from build123d import *

# Parameters (mm, degrees)
CROQUIS1_W              = 60
CROQUIS1_H              = 62
CROQUIS1_R              = 1.5
SALIENTE_EXTRUIR1_DEPTH = 2
REDONDEO1_R             = 4
CROQUIS3_R              = 1.5
CORTAR_EXTRUIR1_DEPTH   = 2


with BuildPart() as part:
    # Croquis1 → Saliente-Extruir1 (new body)
    with BuildSketch(Plane.XY):
        Rectangle(CROQUIS1_W, CROQUIS1_H)
        with Locations((-25, -26)):
            Circle(CROQUIS1_R, mode=Mode.SUBTRACT)
        with Locations((25, -26)):
            Circle(CROQUIS1_R, mode=Mode.SUBTRACT)
        with Locations((25, 26)):
            Circle(CROQUIS1_R, mode=Mode.SUBTRACT)
        with Locations((-25, 26)):
            Circle(CROQUIS1_R, mode=Mode.SUBTRACT)
    extrude(amount=SALIENTE_EXTRUIR1_DEPTH)

    # Redondeo1
    redondeo1_edges = [part.edges().sort_by_distance(p)[0] for p in [
        (-30, -31, 1),
        (-30, 31, 1),
        (30, 31, 1),
        (30, -31, 1),
    ]]
    fillet(redondeo1_edges, radius=REDONDEO1_R)

    # Croquis3 → Cortar-Extruir1 (cut)
    with BuildSketch(Plane.XY.offset(2)):
        with Locations((-10.42, 23.4)):
            Circle(CROQUIS3_R)
        with Locations((-10.42, -23.4)):
            Circle(CROQUIS3_R)
        with Locations((21.5, 0)):
            Circle(CROQUIS3_R)
    extrude(amount=-CORTAR_EXTRUIR1_DEPTH, mode=Mode.SUBTRACT)


solid = part.part
Verification items for the finished model (mm, model axes). Give positions to 0.01 mm unless a question says otherwise; leave off trailing zeros. Order: outer loops, then holes, each group sorted by start corner. A loop starts at its lowest first (then second) coordinate and runs counter-clockwise, first axis right, second up. Notation, with made-up numbers: (39, 63) -> (45, 63) arc R11 cw to (45, 74) -> close; hole circle Ø3 at (-22, 71.5). An arc over 180 degrees is marked (long way). Answer as CSV lines item,"result".
Q1. Sectioned sample at A-A on x = -25. Record the cut outline in (y, z), plus the area to 3 significant figures.
Solutions:
outline,"(-31, 0) -> (-27.5, 0) -> (-27.5, 2) -> (-31, 2) -> close; (-24.5, 0) -> (24.5, 0) -> (24.5, 2) -> (-24.5, 2) -> close; (27.5, 0) -> (31, 0) -> (31, 2) -> (27.5, 2) -> close"
area,"112 mm²"
Q2. Release check for a two-part mould opening along Y. For faces 1 (the cylindrical face through (-28.859, 29.797, 1.014)), 2 (the flat face through (0, 0, 2)), 3 (the cylindrical face through (-10.615, -21.913, 1.014)) record: +Y half, -Y half, draft (parallel to the pull), parting line (faces both ways), or undercut.
Solutions:
face 1,"+Y half"
face 2,"draft"
face 3,"undercut"
Q3. Sectioned sample at C-C on y = 23.4. Record the cut outline in (x, z).
Solutions:
outline,"(-30, 0) -> (-11.92, 0) -> (-11.92, 2) -> (-30, 2) -> close; (-8.92, 0) -> (30, 0) -> (30, 2) -> (-8.92, 2) -> close"
Q4. Scan lines: probe 1 along Y at (x, z) = (25, 1.15); probe 2 along Y at (x, z) = (-10.42, 1); probe 3 along X at (y, z) = (-23.5, 1.25). Record each from-to range of solid material in increasing order.
Solutions:
probe 1,"y = -31 to -27.5, -24.5 to 24.5, 27.5 to 31"
probe 2,"y = -31 to -24.9, -21.9 to 21.9, 24.9 to 31"
probe 3,"x = -30 to -11.92, -8.92 to 30"
Q5. Sectioned sample at D-D on x = 21.5. Record the cut outline in (y, z).
Solutions:
outline,"(-31, 0) -> (-1.5, 0) -> (-1.5, 2) -> (-31, 2) -> close; (1.5, 0) -> (31, 0) -> (31, 2) -> (1.5, 2) -> close"
Q6. Sectioned sample at B-B on y = -26. Record the cut outline in (x, z), plus the area to 3 significant figures.
Solutions:
outline,"(-30, 0) -> (-26.5, 0) -> (-26.5, 2) -> (-30, 2) -> close; (-23.5, 0) -> (23.5, 0) -> (23.5, 2) -> (-23.5, 2) -> close; (26.5, 0) -> (30, 0) -> (30, 2) -> (26.5, 2) -> close"
area,"108 mm²"
